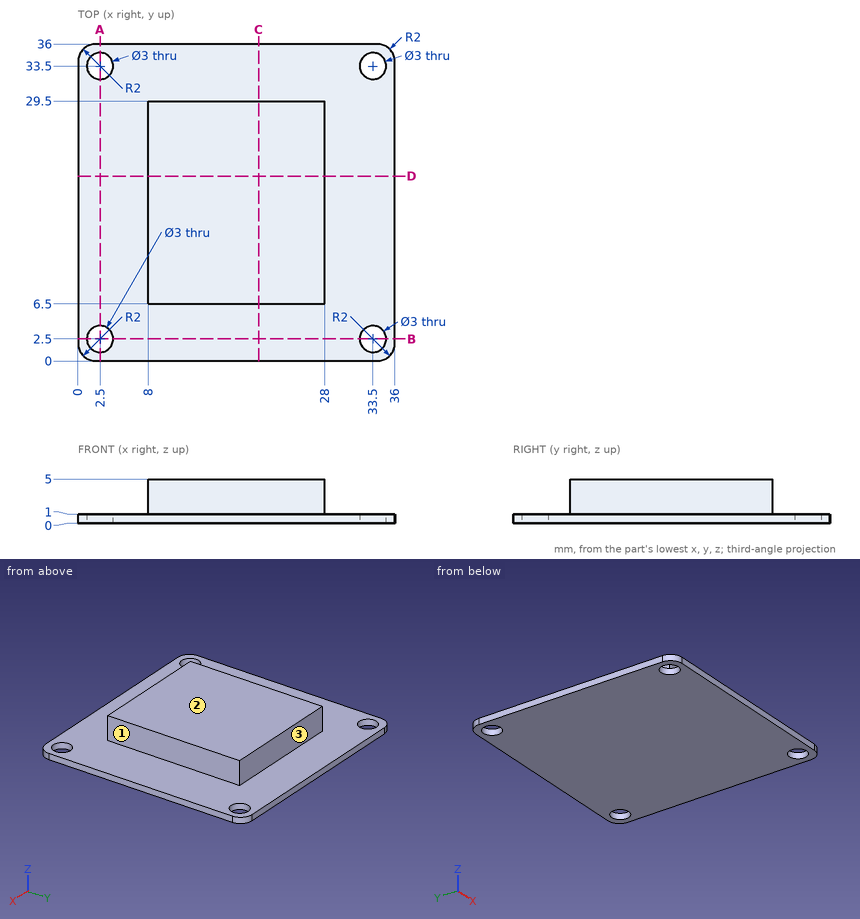
Design review of the part shown in the three views and the two pictorial views. Dimensions are in mm from the part's minimum x, y and z. A direction names the side the tool comes from. Round coordinates to 2 decimals unless told otherwise and drop trailing zeros. Loops run counter-clockwise (first coordinate to the right, second up) from the corner with the lowest first, then second, coordinate; pieces in that order, holes last. Notation, with made-up numbers: (4.5, 74.25) - (18.5, 74.25) arc R13 cw to (18.5, 80.25) - close; hole circle Ø7 at (24, 86.25). An arc over 180 degrees is marked (long way). Write each question's results on one line, items separated by ' | '. Start each with the question number.
Q1. Insertion check: P1, Ø1.2, axis at x = 14.5, z = 3.5, coming from the -Y side; P2, Ø4, axis at x = 2.5, y = 2.5, coming from the +Z side; P3, Ø1.2, axis at y = 19, z = 3.5, coming from the -X side; P4, Ø3, axis at y = 17.5, z = 2, coming from the +X side. Each pin has a flat end and moves straight along its axis. Give the tip position at first contact, or say it passes through.
Q2. Take a section at A-A on x = 2.5. Give the boundary of the cut face in (y, z).
Q3. Take a section at D-D on y = 21. Give the boundary of the cut face in (x, z), plus the area to 3 significant figures.
Q4. Tool access review of the marked faces 1, 2 and 3: name each direction out of +Z, -Z, +X, -X, +Y, -Y from which nothing blocks a thin tool from reaching the whole face with its end or side.
Q5. Wall thickness on line 1 along Y through (x, z) = (33.5, 0.5); line 2 along Z through (x, y) = (16, 4.5); line 3 along X through (y, z) = (15.5, 3.75): over which ranges is each line inside the solid? List them lowest first. Write a range as [from, to].
Q6. Take a section at C-C on x = 20.5. Give the boundary of the cut face in (y, z).
Data:
1) P1: stops at y = 6.5 | P2: stops at z = 1 | P3: stops at x = 8 | P4: stops at x = 36
2) outline: (0, 0) - (1, 0) - (1, 1) - (0, 1) - close; (4, 0) - (32, 0) - (32, 1) - (4, 1) - close; (35, 0) - (36, 0) - (36, 1) - (35, 1) - close
3) outline: (0, 0) - (36, 0) - (36, 1) - (28, 1) - (28, 5) - (8, 5) - (8, 1) - (0, 1) - close | area: 116 mm²
4) face 1: +Z, +X, +Y, -Y | face 2: +Z, +X, -X, +Y, -Y | face 3: +Z, +X, -X, +Y
5) line 1: y = [0, 1], [4, 32], [35, 36] | line 2: z = [0, 1] | line 3: x = [8, 28]
6) outline: (0, 0) - (36, 0) - (36, 1) - (29.5, 1) - (29.5, 5) - (6.5, 5) - (6.5, 1) - (0, 1) - close
